CAD build for the part. Positions are in the model's coordinates, mm. A direction names the side the tool comes from. Round coordinates to 2 decimals unless told otherwise and drop trailing zeros. Order: outer loops, then holes, each group sorted by start corner. A loop starts at its lowest first (then second) coordinate and runs counter-clockwise, first axis right, second up. Notation, with made-up numbers: (60.5, 52) -> (106.5, 52) arc R23 ccw to (106.5, 72) -> close; hole circle Ø3 at (81, 18). An arc over 180 degrees is marked (long way). Return JSON: item names as keys, results as strings. Group by question number.
Q1. Cut at D-D (z = 18). Write the cut outline in (x, y) (3 decimals).
Q2. Which spindle directions (+Z, -Z, +X, -X, +Y, -Y) get a long thin tool onto all of the face, cutting with end or side? Do faces 1 (the flat face through (1.1, 0.4, 28.5)), 2 (the flat face through (4, 8, 20)), 3 (the flat face through (-14.155, 5, 16)), 4 (the flat face through (4, 4, 26)), 5 (the flat face through (-9.3, 6.114, 26.3)). Say none if no direction does.
Q3. Probe line 1 along X through (y, z) = (4.5, 23.5); line 2 along Y through (x, z) = (-7, 7); line 3 along X through (y, z) = (4, 6.5). List the from-to ranges inside material, lowest first.
Q4. Mould opens along X. For faces 6 (the cylindrical face through (-11.546, 6.005, 15.463)), 7 (the flat face through (-10, 5, 0)), 8 (the cylindrical face through (-11.66, 7.1, 26.74)), 9 (the flat face through (-3.155, 1, 13)) say: +X half, -X half, draft (parallel to the pull), parting line (faces both ways), or undercut.
Q5. Cut at C-C (x = 7.5). Write the cut outline in (y, z) (3 decimals).
Q6. Flat gauge pins, fed straight in: pin 1 (1.9 mm diameter, centred on x = -7.5, z = 26, fed in from +Y); pin 2 (1.5 mm diameter, centred on y = 7, z = 14.5, fed in from +X); pin 3 (13 mm diameter, centred on x = 4, z = 11, fed in from +Y); pin 4 (3.5 mm diameter, centred on x = 2, y = 0.5, fed in from -Z). Where does each tip first touch, or does it go through?
Q7. Cut at B-B (y = 5.5). Write the cut outline in (x, z), then the cut area to 3 significant figures.
Q8. Cut at A-A (y = 7.75). Write the cut outline in (x, z), then the cut area to 3 significant figures.
from build123d import *

# Parameters (mm, degrees)
F1_DEPTH      = 20
F2_W          = 7
F2_H          = 20
F3_DEPTH      = 2
F5_DEPTH      = 6
F6_W          = 3
F6_H          = 6
F7_DEPTH      = 25
F8_DEPTH      = 3
F12_DEPTH     = 2
F13_DEPTH     = 11
F14_T4_DEPTH  = 29
F14_T10_DEPTH = 28
F14_T17_DEPTH = 38.2867319519
F14_T24_DEPTH = 39.2867319519
F15_T1_DEPTH  = 61.1449358039
F15_T3_DEPTH  = 60.1449358039
F16_DEPTH     = 1
F17_SIZE      = 6
F20_D         = 2.85
F20_ON_F18_D  = 2.85
F22_DEPTH     = 3
F24_D         = 6.5
F24_DEPTH     = 2
F24_TIP       = 1.9527970118


# Not quite as in the source:
# - a fillet or chamfer that OpenCascade refuses, or shapes differently, is made with other operations: its cross-section is extruded or revolved along the edge and cut away or added


with BuildPart() as f1:
    # F0 (on Top) → F1 (new body)
    with BuildSketch(Plane.XY):
        Polygon((-3.1551690071, 9.1141472052), (-12.1551690071, 9.1141472052), (-12.1551690071, -0.8858527948), (-3.1551690071, -0.8858527948), (-3.1551690071, 2.1141472052), (-9.1551690071, 2.1141472052), (-9.1551690071, 6.1141472052), (-3.1551690071, 6.1141472052), align=None)
    extrude(amount=F1_DEPTH)

    # F2 (on face) → F3 (join)
    with BuildSketch(Plane(origin=(-12.1551690071, 0, 0), x_dir=(0, -1, 0), z_dir=(-1, 0, 0))):
        with Locations((-5.6141472052, 10)):
            Rectangle(F2_W, F2_H)
    extrude(amount=F3_DEPTH)

    # F4 (on face) → F5 (join)
    with BuildSketch(Plane.XY.offset(20)):
        Polygon((-12.1345976368, 9.1141472052), (-12.1551690071, 2.1141472052), (-12.1551690071, -0.8858527948), (-9.1551690071, -0.8858527948), (-9.1551690071, 2.1141472052), (-9.1551690071, 6.1141472052), (-9.1551690071, 9.1141472052), align=None)
    extrude(amount=F5_DEPTH)

    # F6 (on face) → F7 (join)
    with BuildSketch(Plane.YZ.offset(-9.1551690071)):
        with Locations((7.6141472052, 23)):
            Rectangle(F6_W, F6_H)
        with Locations((0.6141472052, 23)):
            Rectangle(F6_W, F6_H)
        Polygon((-0.8858527948, 26), (2.1141472052, 26), (6.1141472052, 26), (9.1141472052, 26), (9.1141472052, 29), (-0.8858527948, 29), align=None)
    extrude(amount=F7_DEPTH)

    # F8 (add): a face of the model
    f8_faces = [f1.faces().sort_by_distance(p)[0] for p in [
        (-10.6515768532, 4.1077318265, 26),
    ]]
    extrude(f8_faces, amount=F8_DEPTH)

    # F9: union 

    # F10: union 

    # F11 (on face) → F12 (join)
    with BuildSketch(Plane.XY.offset(29)):
        Polygon((-12.1345976368, 9.1141472052), (-12.1551690071, 2.1141472052), (15.8448309929, 2.1141472052), (15.8448309929, 9.1141472052), align=None)
    extrude(amount=F12_DEPTH)

    # F4 (on face) → F13 (join)
    with BuildSketch(Plane.XY.offset(20)):
        Polygon((-14.1551690071, 2.1141472052), (-12.1551690071, 2.1141472052), (-12.1345976368, 9.1141472052), (-14.1551690071, 9.1141472052), align=None)
    extrude(amount=F13_DEPTH)

    # F14: chamfer of 4 on 2 edges, made by hand


with BuildPart() as f14_tool2:
    # F14_s3 → F14_t4 (new body)
    with BuildSketch(Plane.XY):
        Polygon((-12.1551690071, -1.8858527948), (-16.1551690071, 2.1141472052), (-12.1551690071, 2.1141472052), align=None)
    extrude(amount=F14_T4_DEPTH)

    split(bisect_by=Plane.XZ.offset(0.8858527948), keep=Keep.BOTTOM)

    split(bisect_by=Plane.YZ.offset(-14.1551690071), keep=Keep.TOP)


with BuildPart() as f1_1:
    add(f1.part)

    # F14_t1: union F14_tool2
    add(f14_tool2.part)


with BuildPart() as f14_tool8:
    # F14_s9 → F14_t10 (new body)
    with BuildSketch(Plane.YZ.offset(-12.1551690071)):
        Polygon((-1.8858527948, 29), (2.1141472052, 33), (2.1141472052, 29), align=None)
    extrude(amount=F14_T10_DEPTH)

    split(bisect_by=Plane.XZ.offset(0.8858527948), keep=Keep.BOTTOM)

    split(bisect_by=Plane.XY.offset(31), keep=Keep.BOTTOM)


with BuildPart() as f1_2:
    add(f1_1.part)

    # F14_t7: union F14_tool8
    add(f14_tool8.part)


with BuildPart() as f14_tool15:
    # F14_s16 → F14_t17 (new body)
    with BuildSketch(Plane.YZ.offset(-22.4419009589)):
        Polygon((-1.8858527948, 29), (2.1141472052, 33), (2.1141472052, 29), align=None)
    extrude(amount=F14_T17_DEPTH)

    split(bisect_by=Plane.XZ.offset(0.8858527948), keep=Keep.BOTTOM)

    split(bisect_by=Plane.YZ.offset(-12.1551690071), keep=Keep.BOTTOM)

    split(bisect_by=Plane.YZ.offset(-14.1551690071), keep=Keep.TOP)

    split(bisect_by=Plane.XY.offset(31), keep=Keep.BOTTOM)


with BuildPart() as f14_tool22:
    # F14_s23 → F14_t24 (new body)
    with BuildSketch(Plane.XY):
        Polygon((-12.1551690071, -1.8858527948), (-16.1551690071, 2.1141472052), (-12.1551690071, 2.1141472052), align=None)
    extrude(amount=F14_T24_DEPTH)

    split(bisect_by=Plane.XZ.offset(0.8858527948), keep=Keep.BOTTOM)

    split(bisect_by=Plane.XY.offset(29), keep=Keep.TOP)

    split(bisect_by=Plane.YZ.offset(-14.1551690071), keep=Keep.TOP)

    split(bisect_by=Plane.XY.offset(31), keep=Keep.BOTTOM)


with BuildPart() as f14_tool15_1:
    add(f14_tool15.part)

    # F14_t29: intersect F14_tool22
    add(f14_tool22.part, mode=Mode.INTERSECT)


with BuildPart() as f1_3:
    add(f1_2.part)

    # F14_t13: union F14_tool15
    add(f14_tool15_1.part)

    # F15: chamfer of 4 x 6 on 2 edges, made by hand

    # F15_s2 → F15_t1 (cut)
    with BuildSketch(Plane.XY.offset(-15.5724679019)):
        Polygon((-9.1551690071, -0.8858527948), (-17.3978096942, 3.3567878923), (-13.1551690071, -0.8858527948), align=None)
    extrude(amount=F15_T1_DEPTH, mode=Mode.SUBTRACT)

    # F15_s4 → F15_t3 (cut)
    with BuildSketch(Plane.YZ.offset(-28.7276369091)):
        Polygon((-0.8858527948, 26), (3.3567878923, 34.2426406871), (-0.8858527948, 30), align=None)
    extrude(amount=F15_T3_DEPTH, mode=Mode.SUBTRACT)

    # F16 (add): a face of the model
    f16_faces = [f1_3.faces().sort_by_distance(p)[0] for p in [
        (15.8448309929, 6.2628078927, 23),
    ]]
    extrude(f16_faces, amount=F16_DEPTH)

    # F17
    f17_edges = [f1_3.edges().sort_by_distance(p)[0] for p in [
        (-3.155169, 0.614147, 0),
        (-3.155169, 7.614147, 0),
        (16.844831, 0.614147, 20),
        (16.844831, 7.614147, 20),
    ]]
    chamfer(f17_edges, length=F17_SIZE)

    # F20 (through all)
    with Locations(Plane(origin=(0, 0, 0), x_dir=(1, 0, 0), z_dir=(0, 0, -1))):
        with Locations((-11.8551690071, -4.6141472052)):
            Hole(F20_D / 2)

    # F20 on F18 (through all)
    with Locations(Plane.YZ.offset(16.8448309929)):
        with Locations((4.6141472052, 30.5)):
            Hole(F20_ON_F18_D / 2)

    # F21 (on face) → F22 (cut)
    with BuildSketch(Plane(origin=(0, 9.1141472052, 0), x_dir=(-1, 0, 0), z_dir=(0, 1, 0))):
        with BuildLine():
            Line((10.2461592647, 27.0909902577), (7.0641787494, 23.9090097423))
            ThreePointArc((7.0641787494, 23.9090097423), (9.5162067299, 23.4212710518), (10.9051690071, 25.5))
            ThreePointArc((10.9051690071, 25.5), (10.7338979552, 26.3610377228), (10.2461592647, 27.0909902577))
        make_face()
        with BuildLine():
            ThreePointArc((10.2461592647, 27.0909902577), (7.0641787494, 27.0909902577), (7.0641787494, 23.9090097423))
            Line((7.0641787494, 23.9090097423), (10.2461592647, 27.0909902577))
        make_face()
    extrude(amount=-F22_DEPTH, mode=Mode.SUBTRACT)

    # F24 (one way)
    with BuildSketch(Plane(origin=(0, 6.1141472052, 0), x_dir=(-1, 0, 0), z_dir=(0, -1, 0))):
        with Locations((8.6551690071, -25.5)):
            Circle(F24_D / 2)
    extrude(amount=-F24_DEPTH, mode=Mode.SUBTRACT)
    with Locations(Plane(origin=(0, 6.1141472052, 0), x_dir=(-1, 0, 0), z_dir=(0, -1, 0))):
        with Locations((8.6551690071, -25.5)):
            with Locations((0, 0, -(F24_DEPTH + F24_TIP / 2))):  # 118° drill point
                Cone(0, F24_D / 2, F24_TIP, mode=Mode.SUBTRACT)


solid = f1_3.part
Solution:
{
 "1": {"outline": "(-14.155, 1.688) -> (-9.155, -0.886) -> (-3.155, -0.886) -> (-3.155, 2.114) -> (-9.155, 2.114) -> (-9.155, 6.114) -> (-3.155, 6.114) -> (-3.155, 9.114) -> (-14.155, 9.114) -> close; hole circle Ø2.85 at (-11.855, 4.614)"},
 "2": {"face 1": "+Z, +X, -X, -Y", "face 2": "-Z, +X, +Y, -Y", "face 3": "+Z, -Z, -X, +Y, -Y", "face 4": "-Z, +X", "face 5": "none"},
 "3": {"line 1": "x = -14.16 to -13.28, -10.43 to -9.16", "line 2": "y = -0.89 to 2.11, 6.11 to 9.11", "line 3": "x = -14.16 to -13.14, -10.57 to -9.16"},
 "4": {"face 6": "undercut", "face 7": "draft", "face 8": "undercut", "face 9": "+X half"},
 "5": {"outline": "(-0.886, 20) -> (2.114, 20) -> (2.114, 26) -> (6.114, 26) -> (6.114, 20) -> (9.114, 20) -> (9.114, 31) -> (5.949, 31) arc R1.425 cw (long way) to (3.28, 31) -> (1.688, 31) -> (-0.886, 26) -> close"},
 "6": {"pin 1": "stops at y = 6.11", "pin 2": "stops at x = -3.16", "pin 3": "passes through", "pin 4": "stops at z = 20"},
 "7": {"outline": "(-14.16, 0) -> (-12.97, 0) -> (-12.97, 29.38) -> (-14.16, 29.38) -> close; (-10.74, 0) -> (-9.16, 0) -> (-9.16, 26) -> (16.84, 26) -> (16.84, 29.38) -> (-10.74, 29.38) -> close", "area": "169 mm²"},
 "8": {"outline": "(-14.16, 0) -> (-9.16, 0) -> (-3.16, 6) -> (-3.16, 20) -> (10.84, 20) -> (16.84, 26) -> (16.84, 31) -> (-14.16, 31) -> close; hole circle Ø6.5 at (-8.66, 25.5)", "area": "492 mm²"}
}
